For this review, take the finished solid that the model builds, in its own axes (mm). Face numbers are marked on the shaded views. A direction names the side the tool comes from. Round coordinates to 2 decimals unless told otherwise and drop trailing zeros. Order: outer loops, then holes, each group sorted by start corner. A loop starts at its lowest first (then second) coordinate and runs counter-clockwise, first axis right, second up. Notation, with made-up numbers: (69.25, 76) - (79.25, 76) arc R18 ccw to (79.25, 90) - close; hole circle Ø5 at (-13, 45). An arc over 180 degrees is marked (long way). Write each question's results on one line, items separated by ' | '. Start each with the question number.
(1) Take a section at D-D, the plane y = 28. Give the boundary of the cut face in (x, z).
(2) Draft analysis for pull direction Z (two halves, no side actions). For the marked faces 1, 2 and 3, state which applies: pulls with the +Z half, pulls with the -Z half, needs draft (parallel to the pull), parting line crosses it, or undercut.
(3) Take a section at A-A, the plane y = 93.5. Give the boundary of the cut face in (x, z).
(4) For the marked faces 4 and 5, list the 3-axis set-ups (+Z, -Z, +X, -X, +Y, -Y) from which the entire face can be reached by the end or side of a thin tool; tool diameter is ignored.
(5) Take a section at C-C, the plane x = 2. Give the boundary of the cut face in (y, z).
(6) Insertion check: pin 1 Ø5 at (x, y) = (23, 108) entering from +Z; pin 2 Ø4 at (y, z) = (107, -15.5) entering from +X; pin 3 Ø6.5 at (y, z) = (75.5, -13.5) entering from +X; pin 4 Ø8 at (y, z) = (32, -14.5) entering from -X. Each pin has a flat end and moves straight along its axis. Give the tip position at first contact, or say it passes through.
(7) For L1, parallel to X at y = 108, z = -12; L2, parallel to Y at x = 5.5, z = -8.5; L3, parallel to X at y = 88, z = -17, list the stretches that pass through material, from the lowest coordinate up. Write a range as from..to.
(8) Take a section at B-B, the plane z = -14.5. Give the boundary of the cut face in (x, y).
```python
from build123d import *

# Parameters (mm, degrees)
BOSS_EXTRUDE1_DEPTH      = 115
FILLET1_R                = 0.5
SHELL1_T                 = -1
SHELL1_THICKNESS_2_DEPTH = 89
SKETCH2_W                = 3
SKETCH2_H                = 4
CUT_EXTRUDE1_DEPTH       = 3


with BuildPart() as part:
    # Sketch1 → Boss-Extrude1 (new body)
    with BuildSketch(Plane(origin=(0, 0, 0), x_dir=(1, 0, 0), z_dir=(0, 1, 0))):
        Polygon((0, 0), (32, 0), (32, 10), (20, 10), (20, 19), (12, 19), (12, 10), (0, 10), align=None)
    extrude(amount=BOSS_EXTRUDE1_DEPTH)

    # Fillet1
    fillet1_edges = [part.edges().sort_by_distance(p)[0] for p in [
        (12, 57.5, -10),
        (12, 57.5, -19),
        (20, 57.5, -19),
        (20, 57.5, -10),
    ]]
    fillet(fillet1_edges, radius=FILLET1_R)

    # Shell1
    shell1_openings = [part.faces().sort_by_distance(p)[0] for p in [
        (16, 115, -6.742495559),
    ]]
    offset(amount=SHELL1_T, openings=shell1_openings)

    # Shell1 thickness 2 face (on inner face of the shell) → Shell1 thickness 2 (add)
    with BuildSketch(Plane(origin=(16, 1, -6.570305912), x_dir=(0, 0, -1), z_dir=(0, -1, 0))):
        with BuildLine():
            ThreePointArc((2.429694088, 4.5), (2.869033916, 3.439339828), (3.929694088, 3))
            Line((3.929694088, 3), (11.429694088, 3))
            Line((11.429694088, 3), (11.429694088, -3))
            Line((11.429694088, -3), (3.929694088, -3))
            ThreePointArc((3.929694088, -3), (2.869033916, -3.439339828), (2.429694088, -4.5))
            Line((2.429694088, -4.5), (2.429694088, -15))
            Line((2.429694088, -15), (-5.570305912, -15))
            Line((-5.570305912, -15), (-5.570305912, 15))
            Line((-5.570305912, 15), (2.429694088, 15))
            Line((2.429694088, 15), (2.429694088, 4.5))
        make_face()
    extrude(amount=-SHELL1_THICKNESS_2_DEPTH)

    # Sketch2 → Cut-Extrude1 (cut)
    with BuildSketch(Plane.XZ):
        with Locations((16, -5)):
            Rectangle(SKETCH2_W, SKETCH2_H)
    extrude(amount=-CUT_EXTRUDE1_DEPTH, mode=Mode.SUBTRACT)


solid = part.part
```
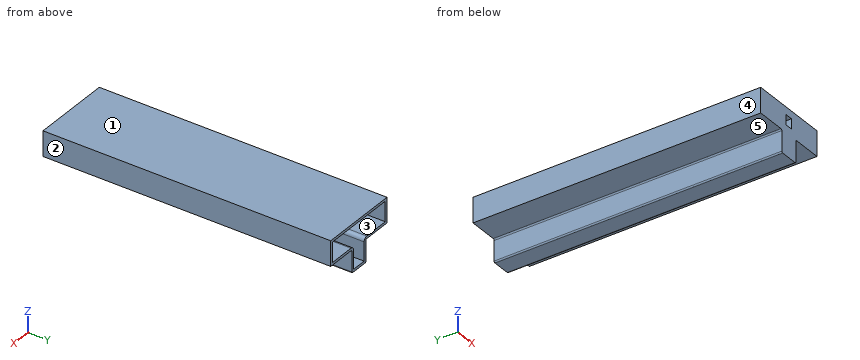
Results below:
1) outline: (0, -10) - (11.5, -10) arc R0.5 cw to (12, -10.5) - (12, -18.5) arc R0.5 ccw to (12.5, -19) - (19.5, -19) arc R0.5 ccw to (20, -18.5) - (20, -10.5) arc R0.5 cw to (20.5, -10) - (32, -10) - (32, 0) - (0, 0) - close
2) face 1: pulls with the +Z half | face 2: needs draft | face 3: undercut
3) outline: (0, -10) - (11.5, -10) arc R0.5 cw to (12, -10.5) - (12, -18.5) arc R0.5 ccw to (12.5, -19) - (19.5, -19) arc R0.5 ccw to (20, -18.5) - (20, -10.5) arc R0.5 cw to (20.5, -10) - (32, -10) - (32, 0) - (0, 0) - close; hole (1, -9) - (11.5, -9) arc R1.5 cw to (13, -10.5) - (13, -18) - (19, -18) - (19, -10.5) arc R1.5 cw to (20.5, -9) - (31, -9) - (31, -1) - (1, -1) - close
4) face 4: +Z, -Z, -X, +Y, -Y | face 5: -Z, -X, +Y, -Y
5) outline: (0, -10) - (115, -10) - (115, -9) - (90, -9) - (90, -1) - (115, -1) - (115, 0) - (0, 0) - close
6) pin 1: stops at z = 0 | pin 2: stops at x = 20 | pin 3: stops at x = 20.07 | pin 4: stops at x = 12
7) L1: x = 12..13, 19..20 | L2: y = 0..90 | L3: x = 12..20
8) outline: (12, 0) - (20, 0) - (20, 115) - (19, 115) - (19, 90) - (13, 90) - (13, 115) - (12, 115) - close
